Autodesk Inventor part; units mm, degrees
ref_plane "YZ Plane" through (0, 0, 0) normal (1, 0, 0) x (0, 1, 0)
ref_plane "XZ Plane" through (0, 0, 0) normal (0, 1, 0) x (-1, 0, 0)
ref_plane "XY Plane" through (0, 0, 0) normal (0, 0, 1) x (1, 0, 0)
ref_plane "Work Plane1" through (-24.4516, 95.9016, -42.078) normal (0, 1, 0) x (-1, 0, 0)
sketch "BaseTop" plane through (-24.4516, 95.9016, -42.078) normal (0, 1, 0) x (-1, 0, 0)
  line L0 (75, 40) -> (-75, 40)
  line L1 (-80, 35) -> (-80, -35)
  line L2 (-75, -40) -> (75, -40)
  line L3 (80, -35) -> (80, 35)
  circle A0 centre (42, 0) radius 6
  arc A1 (80, 35) -> (75, 40) centre (75, 35) ccw
  arc A2 (75, -40) -> (80, -35) centre (75, -35) ccw
  arc A3 (-80, -35) -> (-75, -40) centre (-75, -35) ccw
  arc A4 (-75, 40) -> (-80, 35) centre (-75, 35) ccw
  circle A5 centre (42, 0) radius 19
  point P0 (-24.4516, 42.078)
  dimension "d1" = 12
  dimension "d2" = 5
  dimension "d15" = 38
extrude "Extrusion1" add sketch "BaseTop" along normal blind 7.5 contours A1 L3 A2 L2 A3 L1 A4 L0 | A0 | A5
extrude "Extrusion6" cut sketch "BaseTop" along normal blind 2 contours A0 | A5
sketch "Sketch6" plane through (-24.4516, 103.4016, -42.078) normal (0, 1, 0) x (1, 0, 0)
  circle A0 centre (-42, 0) radius 15
  point P0 (24.4516, -42.078)
  dimension "d20" = 30
extrude "Extrusion7" cut sketch "Sketch6" against normal blind 3
extrude "Extrusion8" cut sketch "BaseTop" along normal through all contours A0
properties part number "BaseTop"
Verification items for the finished model (mm, model axes). A direction names the side the tool comes from. Coordinates: 2 decimals unless noted, no trailing zeros. Loops run counter-clockwise (first coordinate to the right, second up) from the corner with the lowest first, then second, coordinate; pieces in that order, holes last. Notation, with made-up numbers: (40, 25) - (54, 25) arc R25 ccw to (54, 59) - close; hole circle Ø7 at (-40, -12.75). An arc over 180 degrees is marked (long way). Return JSON: item names as keys, results as strings.
1. Mould release check, pull along Z, two halves, no side actions. Record for faces 4 (the cylindrical face through (-102.948, 99.599, -3.504)), 5 (the cylindrical face through (-71.994, 99.134, -39.78)), 6 (the flat face through (55.548, 100, -42)): +Z half, -Z half, draft (parallel to the pull), parting line (faces both ways), or undercut.
Established:
{"face 4": "+Z half", "face 5": "undercut", "face 6": "draft"}
2. Section check C-C, the plane x = -57. Record the boundary of the cut face in (y, z).
Established:
{"outline": "(95.9, -82.08) - (103.4, -82.08) - (103.4, -53.73) - (100.4, -53.73) - (100.4, -30.43) - (103.4, -30.43) - (103.4, -2.08) - (95.9, -2.08) - (95.9, -25.6) - (97.9, -25.6) - (97.9, -58.56) - (95.9, -58.56) - close"}
3. Go/stop test with flat-tipped pins: pin 1 (15.5 mm diameter, centred on x = -66.45, z = -42.08, fed in from -Y); pin 2 (18 mm diameter, centred on x = -66.45, z = -42.08, fed in from +Y); pin 3 (24 mm diameter, centred on x = -59.5, z = -47.5, fed in from +Y). Record where each tip stops, or that it passes through.
Established:
{"pin 1": "stops at y = 97.9", "pin 2": "stops at y = 100.4", "pin 3": "stops at y = 103.4"}
4. Section check B-B, the plane x = -77. Record the boundary of the cut face in (y, z).
Established:
{"outline": "(95.9, -82.08) - (103.4, -82.08) - (103.4, -52.74) - (100.4, -52.74) - (100.4, -31.41) - (103.4, -31.41) - (103.4, -2.08) - (95.9, -2.08) - (95.9, -26.28) - (97.9, -26.28) - (97.9, -57.88) - (95.9, -57.88) - close"}
5. Tool access check on faces 1 (the cylindrical face through (54.045, 99.599, -80.652)), 2 (the cylindrical face through (-51.37, 96.89, -30.52)), 3 (the cylindrical face through (-58.388, 101.923, -54.726)). Record the directions out of +Z, -Z, +X, -X, +Y, -Y that give a thin tool (end or side, any length) a straight path to the whole face; none if there is none.
Established:
{"face 1": "-Z, +X, +Y, -Y", "face 2": "-Y", "face 3": "+Y"}
6. Thickness scan on L1, parallel to X at y = 101, z = -55.5; L2, parallel to Z at x = -82, y = 97.25; L3, parallel to X at y = 102.5, z = -33. Record the ranges inside material, lowest first.
Established:
{"L1": "x = -104.45 to -73.15, -59.75 to 55.55", "L2": "z = -82.08 to -53, -31.16 to -2.08", "L3": "x = -104.45 to -78.39, -54.51 to 55.55"}
7. Section check A-A, the plane z = -44. Record the boundary of the cut face in (x, y), then the cut area to 3 significant figures.
Established:
{"outline": "(-104.45, 95.9) - (-85.35, 95.9) - (-85.35, 97.9) - (-72.14, 97.9) - (-72.14, 100.4) - (-81.33, 100.4) - (-81.33, 103.4) - (-104.45, 103.4) - close; (-60.77, 97.9) - (-47.55, 97.9) - (-47.55, 95.9) - (55.55, 95.9) - (55.55, 103.4) - (-51.58, 103.4) - (-51.58, 100.4) - (-60.77, 100.4) - close", "area": "1,010 mm2"}
